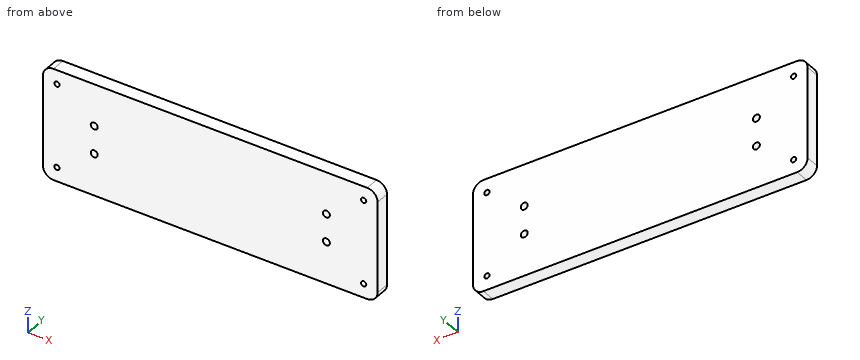
```python
from build123d import *

# Parameters (mm, degrees)
F0_W     = 304.8
F0_H     = 101.6
F1_DEPTH = 12.7
F2_R     = 9.525
F4_D     = 4.7752
F6_D     = 6.35


with BuildPart() as f1:
    # F0 (on Front) → F1 (new body)
    with BuildSketch(Plane.XZ):
        with Locations((152.4, 50.8)):
            Rectangle(F0_W, F0_H)
    extrude(amount=F1_DEPTH)

    # F2
    f2_edges = [f1.edges().sort_by_distance(p)[0] for p in [
        (0, -6.35, 101.6),
        (304.8, -6.35, 101.6),
        (304.8, -6.35, 0),
        (0, -6.35, 0),
    ]]
    fillet(f2_edges, radius=F2_R)

    # F4 (through all)
    with Locations(Plane.XZ.offset(12.7)):
        with Locations((12.7, 88.9), (12.7, 12.7), (292.1, 12.7), (292.1, 88.9)):
            Hole(F4_D / 2)

    # F6 (through all)
    with Locations(Plane.XZ.offset(12.7)):
        with Locations((46.666421, 63.5), (46.666421, 38.1), (258.133579, 63.5), (258.133579, 38.1)):
            Hole(F6_D / 2)


solid = f1.part
```
Input: part model. Units: mm. Frame: model coordinates. Give positions to 0.01 mm unless a question says otherwise; leave off trailing zeros. Loops run counter-clockwise (first coordinate to the right, second up) from the corner with the lowest first, then second, coordinate; pieces in that order, holes last. Notation, with made-up numbers: M 13.5,62 L 63.5,62 A20 ccw 63.5,70 Z; hole C 40,25.25 d7. An arc over 180 degrees is marked long. Answer as CSV lines item,"result". Start each with the question number.
1. Line query: L1, parallel to Z at x = 12.7, y = -4; L2, parallel to Z at x = 258, y = -4.5; L3, parallel to X at y = -6.5, z = 14. Output: solid intervals per line, ascending.
2. Section A-A on z = 38.1. Return loops of the section in (x, y).
3. Pin query (flat end, axial travel): P1, Ø4, axis at x = 12.7, z = 88.9, coming from the +Y side. Return the tip coordinate at first contact, or that it passes through.
Computed values:
1,L1,"z = 0 to 10.31, 15.09 to 86.51, 91.29 to 101.6"
1,L2,"z = 0 to 34.93, 41.27 to 60.33, 66.67 to 101.6"
1,L3,"x = 0 to 10.7, 14.7 to 290.1, 294.1 to 304.8"
2,outline,"M 0,-12.7 L 43.49,-12.7 L 43.49,0 L 0,0 Z; M 49.84,-12.7 L 254.96,-12.7 L 254.96,0 L 49.84,0 Z; M 261.31,-12.7 L 304.8,-12.7 L 304.8,0 L 261.31,0 Z"
3,P1,"passes through"
